Input: part model. Units: mm. Frame: model coordinates. Face numbers are marked on the shaded views. A direction names the side the tool comes from. Give positions to 0.01 mm unless a question says otherwise; leave off trailing zeros. Loops run counter-clockwise (first coordinate to the right, second up) from the corner with the lowest first, then second, coordinate; pieces in that order, holes last. Notation, with made-up numbers: (36.5, 38.5) -> (51.5, 38.5) arc R15 cw to (51.5, 50.5) -> close; hole circle Ø11 at (6, 47). An arc over 180 degrees is marked (long way). Answer as a JSON object with one key per item and string values. Group by question number.
```python
from build123d import *

# Parameters (mm, degrees)
SKETCH1_W           = 60
SKETCH1_H           = 54
BOSS_EXTRUDE1_DEPTH = 38
SKETCH2_W           = 44
SKETCH2_H           = 52
CUT_EXTRUDE1_DEPTH  = 19
SKETCH3_W           = 35
SKETCH3_H           = 52
CUT_EXTRUDE2_DEPTH  = 18
SKETCH4_W           = 6
SKETCH4_H           = 10
CUT_EXTRUDE3_DEPTH  = 38
SKETCH5_W           = 14
SKETCH5_H           = 52
CUT_EXTRUDE5_DEPTH  = 15
SKETCH6_W           = 13
SKETCH6_H           = 52
CUT_EXTRUDE6_DEPTH  = 4
SKETCH8_W           = 15
SKETCH8_H           = 13
CUT_EXTRUDE7_DEPTH  = 6
SKETCH10_W          = 13
SKETCH10_H          = 5
CUT_EXTRUDE8_DEPTH  = 6
SKETCH11_W          = 4
SKETCH11_H          = 5
CUT_EXTRUDE9_DEPTH  = 3
SKETCH12_W          = 5
SKETCH12_H          = 2
CUT_EXTRUDE10_DEPTH = 13
CUT_EXTRUDE11_DEPTH = 1
SKETCH14_W          = 13
SKETCH14_H          = 1
BOSS_EXTRUDE2_DEPTH = 4
SKETCH15_W          = 13
SKETCH15_H          = 1
BOSS_EXTRUDE3_DEPTH = 4
CUT_EXTRUDE12_DEPTH = 1
CUT_EXTRUDE13_DEPTH = 1


with BuildPart() as part:
    # Sketch1 → Boss-Extrude1 (new body)
    with BuildSketch(Plane(origin=(0, 0, 0), x_dir=(1, 0, 0), z_dir=(0, 1, 0))):
        with Locations((-83.874465942, -33.946435202)):
            Rectangle(SKETCH1_W, SKETCH1_H)
    extrude(amount=BOSS_EXTRUDE1_DEPTH)

    # Sketch2 → Cut-Extrude1 (cut)
    with BuildSketch(Plane(origin=(0, 38, 0), x_dir=(1, 0, 0), z_dir=(0, 1, 0))):
        with Locations((-76.874465942, -33.946435202)):
            Rectangle(SKETCH2_W, SKETCH2_H)
    extrude(amount=-CUT_EXTRUDE1_DEPTH, mode=Mode.SUBTRACT)

    # Sketch3 → Cut-Extrude2 (cut)
    with BuildSketch(Plane(origin=(0, 0, 0), x_dir=(-1, 0, 0), z_dir=(0, -1, 0))):
        with Locations((95.374465942, -33.946435202)):
            Rectangle(SKETCH3_W, SKETCH3_H)
    extrude(amount=-CUT_EXTRUDE2_DEPTH, mode=Mode.SUBTRACT)

    # Sketch4 → Cut-Extrude3 (cut)
    with BuildSketch(Plane(origin=(0, 18, 0), x_dir=(-1, 0, 0), z_dir=(0, -1, 0))):
        with Locations((108.874465942, -34.946435202)):
            Rectangle(SKETCH4_W, SKETCH4_H)
    extrude(amount=-CUT_EXTRUDE3_DEPTH, mode=Mode.SUBTRACT)

    # Sketch5 → Cut-Extrude5 (cut)
    with BuildSketch(Plane(origin=(0, 38, 0), x_dir=(1, 0, 0), z_dir=(0, 1, 0))):
        with Locations((-105.874465942, -33.946435202)):
            Rectangle(SKETCH5_W, SKETCH5_H)
    extrude(amount=-CUT_EXTRUDE5_DEPTH, mode=Mode.SUBTRACT)

    # Sketch6 → Cut-Extrude6 (cut)
    with BuildSketch(Plane(origin=(0, 23, 0), x_dir=(1, 0, 0), z_dir=(0, 1, 0))):
        with Locations((-106.374465942, -33.946435202)):
            Rectangle(SKETCH6_W, SKETCH6_H)
    extrude(amount=-CUT_EXTRUDE6_DEPTH, mode=Mode.SUBTRACT)

    # Sketch8 → Cut-Extrude7 (cut)
    with BuildSketch(Plane(origin=(0, 0, 0), x_dir=(-1, 0, 0), z_dir=(0, -1, 0))):
        with Locations((65.874465942, -17.946435202)):
            Rectangle(SKETCH8_W, SKETCH8_H)
    extrude(amount=-CUT_EXTRUDE7_DEPTH, mode=Mode.SUBTRACT)

    # Sketch10 → Cut-Extrude8 (cut)
    with BuildSketch(Plane(origin=(-73.374465942, 0, 0), x_dir=(0, 0, -1), z_dir=(1, 0, 0))):
        with Locations((-17.946435202, 3.5)):
            Rectangle(SKETCH10_W, SKETCH10_H)
    extrude(amount=-CUT_EXTRUDE8_DEPTH, mode=Mode.SUBTRACT)

    # Sketch11 → Cut-Extrude9 (cut)
    with BuildSketch(Plane.XZ):
        with Locations((-65.874465942, 48.446435202)):
            Rectangle(SKETCH11_W, SKETCH11_H)
    extrude(amount=-CUT_EXTRUDE9_DEPTH, mode=Mode.SUBTRACT)

    # Sketch12 → Cut-Extrude10 (cut)
    with BuildSketch(Plane(origin=(-67.874465942, 0, 0), x_dir=(0, 0, -1), z_dir=(1, 0, 0))):
        with Locations((-48.446435202, 2)):
            Rectangle(SKETCH12_W, SKETCH12_H)
    extrude(amount=-CUT_EXTRUDE10_DEPTH, mode=Mode.SUBTRACT)

    # Sketch13 → Cut-Extrude11 (cut)
    with BuildSketch(Plane.ZY.offset(113.874465942)):
        with BuildLine():
            Line((32.733045904, 15), (32.733045904, 22))
            ThreePointArc((32.733045904, 22), (35.233045904, 24.5), (37.733045904, 22))
            Line((37.733045904, 22), (37.733045904, 15))
            ThreePointArc((37.733045904, 15), (35.233045904, 12.5), (32.733045904, 15))
        make_face()
    extrude(amount=-CUT_EXTRUDE11_DEPTH, mode=Mode.SUBTRACT)

    # Sketch14 → Boss-Extrude2 (add)
    with BuildSketch(Plane(origin=(0, 19, 0), x_dir=(1, 0, 0), z_dir=(0, 1, 0))):
        with Locations((-106.374465942, -40.446435202)):
            Rectangle(SKETCH14_W, SKETCH14_H)
    extrude(amount=BOSS_EXTRUDE2_DEPTH)

    # Sketch15 → Boss-Extrude3 (add)
    with BuildSketch(Plane(origin=(0, 19, 0), x_dir=(1, 0, 0), z_dir=(0, 1, 0))):
        with Locations((-106.374465942, -29.446435202)):
            Rectangle(SKETCH15_W, SKETCH15_H)
    extrude(amount=BOSS_EXTRUDE3_DEPTH)

    # Sketch16 → Cut-Extrude12 (cut)
    with BuildSketch(Plane(origin=(0, 19, 0), x_dir=(1, 0, 0), z_dir=(0, 1, 0))):
        with BuildLine():
            Line((-64.874465942, -54.946435202), (-88.874465942, -54.946435202))
            ThreePointArc((-88.874465942, -54.946435202), (-92.409999848, -53.481969108), (-93.874465942, -49.946435202))
            Line((-93.874465942, -49.946435202), (-93.874465942, -41.446435202))
            ThreePointArc((-93.874465942, -41.446435202), (-92.409999848, -37.910901296), (-88.874465942, -36.446435202))
            Line((-88.874465942, -36.446435202), (-64.874465942, -36.446435202))
            ThreePointArc((-64.874465942, -36.446435202), (-61.338932037, -37.910901296), (-59.874465942, -41.446435202))
            Line((-59.874465942, -41.446435202), (-59.874465942, -49.946435202))
            ThreePointArc((-59.874465942, -49.946435202), (-61.338932037, -53.481969108), (-64.874465942, -54.946435202))
        make_face()
        with BuildLine():
            Line((-88.874465942, -31.446435202), (-64.874465942, -31.446435202))
            ThreePointArc((-64.874465942, -31.446435202), (-61.338932037, -29.981969108), (-59.874465942, -26.446435202))
            Line((-59.874465942, -26.446435202), (-59.874465942, -17.946435202))
            ThreePointArc((-59.874465942, -17.946435202), (-61.338932037, -14.410901296), (-64.874465942, -12.946435202))
            Line((-64.874465942, -12.946435202), (-88.874465942, -12.946435202))
            ThreePointArc((-88.874465942, -12.946435202), (-92.409999848, -14.410901296), (-93.874465942, -17.946435202))
            Line((-93.874465942, -17.946435202), (-93.874465942, -26.446435202))
            ThreePointArc((-93.874465942, -26.446435202), (-92.409999848, -29.981969108), (-88.874465942, -31.446435202))
        make_face()
    extrude(amount=-CUT_EXTRUDE12_DEPTH, mode=Mode.SUBTRACT)

    # Sketch17 → Cut-Extrude13 (cut)
    with BuildSketch(Plane(origin=(0, 19, 0), x_dir=(1, 0, 0), z_dir=(0, 1, 0))):
        with BuildLine():
            Line((-104.874465942, -57.446435202), (-107.874465942, -57.446435202))
            ThreePointArc((-107.874465942, -57.446435202), (-109.642232895, -56.714202155), (-110.374465942, -54.946435202))
            Line((-110.374465942, -54.946435202), (-110.374465942, -45.946435202))
            ThreePointArc((-110.374465942, -45.946435202), (-109.642232895, -44.178668249), (-107.874465942, -43.446435202))
            Line((-107.874465942, -43.446435202), (-104.874465942, -43.446435202))
            ThreePointArc((-104.874465942, -43.446435202), (-103.10669899, -44.178668249), (-102.374465942, -45.946435202))
            Line((-102.374465942, -45.946435202), (-102.374465942, -54.946435202))
            ThreePointArc((-102.374465942, -54.946435202), (-103.10669899, -56.714202155), (-104.874465942, -57.446435202))
        make_face()
        with BuildLine():
            Line((-104.874465942, -26.446435202), (-107.874465942, -26.446435202))
            ThreePointArc((-107.874465942, -26.446435202), (-109.642232895, -25.714202155), (-110.374465942, -23.946435202))
            Line((-110.374465942, -23.946435202), (-110.374465942, -12.946435202))
            ThreePointArc((-110.374465942, -12.946435202), (-109.642232895, -11.178668249), (-107.874465942, -10.446435202))
            Line((-107.874465942, -10.446435202), (-104.874465942, -10.446435202))
            ThreePointArc((-104.874465942, -10.446435202), (-103.10669899, -11.178668249), (-102.374465942, -12.946435202))
            Line((-102.374465942, -12.946435202), (-102.374465942, -23.946435202))
            ThreePointArc((-102.374465942, -23.946435202), (-103.10669899, -25.714202155), (-104.874465942, -26.446435202))
        make_face()
    extrude(amount=-CUT_EXTRUDE13_DEPTH, mode=Mode.SUBTRACT)


solid = part.part
```
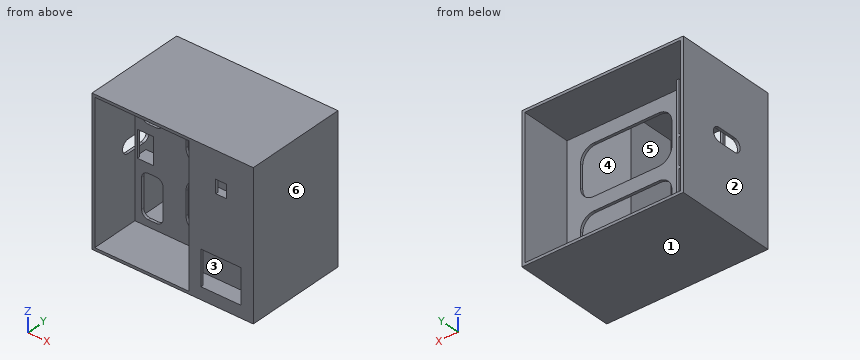
Q1. Section D-D on y = 9.5. Return the cut outline in (x, z), then the cut area to 3 significant figures.
Q2. Ray query, probe 1 along X at (y, z) = (25.5, 57.5); probe 2 along Z at (x, y) = (-91.5, 32.5); probe 3 along X at (y, z) = (22.5, 44.5). Return the intervals inside material, ascending.
Q3. Section C-C on x = -92. Return the cut outline in (y, z), then the cut area to 3 significant figures.
Q4. Pull-direction query (Z, two-part tool) for the marked faces 1, 2 and 3; classes: +Z half, -Z half, draft (parallel to the pull), parting line (faces both ways), or undercut.
Q5. Section A-A on x = -75.5. Return the cut outline in (y, z).
Q6. Pin query (flat end, axial travel): pin 1 Ø14.5 at (x, z) = (-69.5, 21) entering from +Y; pin 2 Ø6 at (x, z) = (-82, 32) entering from +Y. Return the tip coordinate at first contact, or that it passes through.
Q7. Set-up query: the marked faces 4, 5 and 6. Return all of +Z, -Z, +X, -X, +Y, -Y with unobstructed straight access to the full face (end or side cutting, diameter ignored); none if empty.
Q8. Section B-B on y = 25.5. Return the cut outline in (x, z).
Numbers:
{
 "1": {"outline": "(-113.87, 6.95) -> (-53.87, 6.95) -> (-53.87, 60.95) -> (-113.87, 60.95) -> close; hole (-112.87, 7.95) -> (-77.87, 7.95) -> (-77.87, 59.95) -> (-112.87, 59.95) -> close", "area": "1,420 mm²"},
 "2": {"probe 1": "x = -113.87 to -112.87, -54.87 to -53.87", "probe 2": "z = 6.95 to 7.95, 59.95 to 60.95", "probe 3": "x = -113.87 to -112.87, -99.87 to -98.87, -54.87 to -53.87"},
 "3": {"outline": "(0, 6.95) -> (38, 6.95) -> (38, 7.95) -> (19, 7.95) -> (19, 14.04) -> (18, 14.04) -> (18, 7.95) -> (0, 7.95) -> close; (0, 59.95) -> (18, 59.95) -> (18, 53.85) -> (19, 53.85) -> (19, 59.95) -> (38, 59.95) -> (38, 60.95) -> (0, 60.95) -> close; (18, 30.35) -> (19, 30.35) -> (19, 37.54) -> (18, 37.54) -> close", "area": "95.4 mm²"},
 "4": {"face 1": "-Z half", "face 2": "draft", "face 3": "undercut"},
 "5": {"outline": "(0, 6.95) -> (38, 6.95) -> (38, 7.95) -> (19, 7.95) -> (19, 12.95) -> (18, 12.95) -> (18, 31.45) -> (19, 31.45) -> (19, 36.45) -> (18, 36.45) -> (18, 54.95) -> (19, 54.95) -> (19, 59.95) -> (38, 59.95) -> (38, 60.95) -> (0, 60.95) -> close; hole (1, 11.45) -> (6, 11.45) -> (6, 24.45) -> (1, 24.45) -> close; hole (1, 45.95) -> (3, 45.95) -> (3, 50.95) -> (1, 50.95) -> close"},
 "6": {"pin 1": "stops at y = 18", "pin 2": "stops at y = 19"},
 "7": {"face 4": "+Y", "face 5": "-Y", "face 6": "+Z, -Z, +X, +Y, -Y"},
 "8": {"outline": "(-113.87, 6.95) -> (-53.87, 6.95) -> (-53.87, 60.95) -> (-113.87, 60.95) -> close; hole (-112.87, 7.95) -> (-54.87, 7.95) -> (-54.87, 59.95) -> (-112.87, 59.95) -> close"}
}
